Autodesk Inventor part; units mm, degrees
ref_plane "Plano de trabajo1" through (-16.5, -8, 30) normal (0, 0, 1) x (1, 0, 0)
ref_plane "YZ Plane" through (0, 0, 0) normal (1, 0, 0) x (0, 1, 0)
ref_plane "XZ Plane" through (0, 0, 0) normal (0, 1, 0) x (-1, 0, 0)
sketch "Boceto1" plane through (0, 0, 0) normal (0, 0, 1) x (1, 0, 0)
  circle A0 centre (-8.5, 0) radius 8.65
  circle A1 centre (-8.5, -11.5) radius 1.75
  circle A2 centre (-8.5, 11.5) radius 1.75
  circle A3 centre (-8.5, 0) radius 14.5
  circle A4 centre (-8.5, 0) radius 14.5
  circle A5 centre (-8.5, 0) radius 9.5
  circle A6 centre (-8.5, -11.5) radius 2.25
  circle A7 centre (-8.5, 11.5) radius 2.25
  point P0 (0, 0)
  dimension "d0" = 17.3
  dimension "d1" = 3.5
  dimension "d2" = 3.5
  dimension "d3" = 19
  dimension "d4" = 4.5
  dimension "d5" = 4.5
sketch "Boceto2" plane through (0, 0, 0) normal (0, 0, 1) x (1, 0, 0)
  arc A0 (6.4812, 0.75) -> (6.4812, -0.75) centre (-8.5, 0) ccw
  circle A1 centre (-8.5, 0) radius 15
  point P0 (0, 0)
  point P1 (6.4812, -0.75)
  point P2 (6.4812, 0.75)
extrude "Extrusión1" add sketch "Boceto2" along normal blind 3.5
sketch "Boceto3" plane through (-8.5, 0, 3.5) normal (0, 0, 1) x (1, 0, 0)
  circle A0 centre (0, -11.5) radius 1.75
  circle A1 centre (0, -11.5) radius 2.25
  circle A2 centre (0, 0) radius 9.5
  circle A3 centre (0, 0) radius 8.65
  circle A4 centre (0, 11.5) radius 2.25
  circle A5 centre (0, 11.5) radius 1.75
  point P0 (8.5, 0)
  point P1 (0.9357, 9.4538)
  point P2 (-0.9357, 9.4538)
  point P3 (-0.9357, -9.4538)
  point P4 (0.9357, -9.4538)
sketch "Boceto4" plane through (-8.5, 0, 3.5) normal (0, 0, 1) x (1, 0, 0)
  circle A0 centre (0, 0) radius 5
  point P0 (8.5, 0)
  dimension "d8" = 10
extrude "Extrusión2" cut sketch "Boceto4" against normal blind 10
ref_plane "Plano de trabajo1" through (-16.5, -8, 30) normal (0, 0, 1) x (1, 0, 0)
extrude "Extrusión3" add sketch "Boceto3" along normal up to surface (26.5 mm away) contours A1 A2 A4
extrude "Extrusión4" cut sketch "Boceto1" along normal blind 10 contours A1 | A2
sketch "Boceto5" plane through (-8.5, 11.5, 30) normal (0, 0, 1) x (1, 0, 0)
  arc A0 (0.9357, -20.9538) -> (0.9357, -2.0462) centre (0, -11.5) ccw
  arc A1 (-0.9357, -2.0462) -> (-0.9357, -20.9538) centre (0, -11.5) ccw
  arc A2 (-0.9357, -2.0462) -> (0.9357, -2.0462) centre (0, 0) ccw
  arc A3 (0.9357, -20.9538) -> (-0.9357, -20.9538) centre (0, -23) ccw
  circle A4 centre (0, -11.5) radius 8.65
  point P0 (8.5, -11.5)
extrude "Extrusión5" add sketch "Boceto5" along normal blind 2
sketch "Boceto6" plane through (-8.5, 11.5, 32) normal (0, 0, 1) x (1, 0, 0)
  circle A0 centre (0, -11.5) radius 15
  circle A1 centre (0, -11.5) radius 5
  circle A2 centre (0, -11.5) radius 5
  point P0 (8.5, -11.5)
extrude "Extrusión6" add sketch "Boceto6" along normal blind 3
sketch "Boceto7" plane through (-8.5, 0, 0) normal (0, 0, -1) x (-1, 0, 0)
  circle A0 centre (0, 0) radius 5
  circle A1 centre (0, 0) radius 8.65
  point P0 (-8.5, 0)
  dimension "d19" = 17.3
extrude "Extrusión7" cut sketch "Boceto7" against normal blind 10 contours A0 | A1
properties part number "TeceraParte"
Geometry check sheet. Reference: the model listing, model coordinates, mm. A direction names the side the tool comes from. Give positions to 0.01 mm unless a question says otherwise; leave off trailing zeros. Order: outer loops, then holes, each group sorted by start corner. A loop starts at its lowest first (then second) coordinate and runs counter-clockwise, first axis right, second up. Notation, with made-up numbers: (-5.5, 24) - (-0.5, 24) arc R25 ccw to (-0.5, 57) - close; hole circle Ø2 at (45, -39). An arc over 180 degrees is marked (long way). Write item = value, one per line. Start each with the question number.
1) Gauge pin test, flat ends, axial feed: pin 1 Ø2 at (x, z) = (-16, 9.5) entering from +Y; pin 2 Ø4 at (x, z) = (-2.5, 7) entering from +Y; pin 3 Ø10 at (x, y) = (-20.5, 10.5) entering from -Z; pin 4 Ø3 at (y, z) = (9, 20.5) entering from +X. Record the tip position at first contact, or that the pin passes through.
2) Section check A-A (x = -8.5). Enter the section's corners in (y, z), then the cut area to 3 significant figures.
3) Section check D-D (y = -3). Enter the section's corners in (x, z).
4) Draft check along Y on faces 4 (the cylindrical face through (-7.6, 10, 1.7)), 5 (the cylindrical face through (6.5, 0, 1.7)), 6 (the flat face through (-9, -10, 32)). Enter one of: released by +Y, released by -Y, zero draft, split by the parting line, or undercut.
5) Access from +Z, -Z, +X, -X, +Y, -Y to the whole of each face (thin tool, end or side, straight path). Record for faces 1 (the flat face through (1.3, 0.2, 3.5)), 2 (the cylindrical face through (-7.6, -13, 1.7)), 3 (the flat face through (-12, 4, 35)).
6) Section check C-C (z = 29). Enter the section's corners in (x, y), then the cut area to 3 significant figures.
7) Scan lines: L1, parallel to Y at x = -8.5, z = 1.4; L2, parallel to Y at x = -8.5, z = 20; L3, parallel to Z at x = 5.25, y = -3.25. Record each from-to range of solid material in increasing order.
8) Section check B-B (y = -11.5). Enter the section's corners in (x, z), then the cut area to 3 significant figures.
Geometry check:
q1.pin_1 = 6.93
q1.pin_2 = 8.62
q1.pin_3 = 0
q1.pin_4 = -2.67
q2.outline = (-15, 0) - (-13.25, 0) - (-13.25, 3.5) - (-15, 3.5) - close; (-15, 32) - (-9.25, 32) - (-9.25, 3.5) - (-9.75, 3.5) - (-9.75, 0) - (-8.65, 0) - (-8.65, 32) - (-5, 32) - (-5, 35) - (-15, 35) - close; (5, 32) - (8.65, 32) - (8.65, 0) - (9.75, 0) - (9.75, 3.5) - (9.25, 3.5) - (9.25, 32) - (15, 32) - (15, 35) - (5, 35) - close; (13.25, 0) - (15, 0) - (15, 3.5) - (13.25, 3.5) - close
q2.area = 114 mm2
q3.outline = (-23.2, 0) - (-16.61, 0) - (-16.61, 32) - (-12.5, 32) - (-12.5, 35) - (-23.2, 35) - (-23.2, 32) - (-17.51, 32) - (-17.51, 3.5) - (-23.2, 3.5) - close; (-4.5, 32) - (-0.39, 32) - (-0.39, 0) - (6.2, 0) - (6.2, 3.5) - (0.51, 3.5) - (0.51, 32) - (6.2, 32) - (6.2, 35) - (-4.5, 35) - close
q4.face_4 = undercut
q4.face_5 = split by the parting line
q4.face_6 = zero draft
q5.face_1 = none
q5.face_2 = -Z
q5.face_3 = +Z, +X, -X, +Y, -Y
q6.outline = (-9.44, -9.45) arc R2.25 cw to (-7.56, -9.45) arc R9.5 ccw to (-7.56, 9.45) arc R2.25 cw to (-9.44, 9.45) arc R9.5 ccw to start; hole circle Ø17.3 at (-8.5, 0)
q6.area = 47.8 mm2
q7.L1 = -15 to -13.25, -9.75 to -8.65, 8.65 to 9.75, 13.25 to 15
q7.L2 = -9.25 to -8.65, 8.65 to 9.25
q7.L3 = 0 to 3.5, 32 to 35
q8.outline = (-18.13, 0) - (-10.25, 0) - (-10.25, 3.5) - (-18.13, 3.5) - close; (-18.13, 32) - (1.13, 32) - (1.13, 35) - (-18.13, 35) - close; (-6.75, 0) - (1.13, 0) - (1.13, 3.5) - (-6.75, 3.5) - close
q8.area = 113 mm2
